Check sheet for the modelled part. Datum: model origin and axes. Units: mm. Face numbers are marked on the shaded views. A direction names the side the tool comes from. Coordinates: 2 decimals unless noted, no trailing zeros. Order: outer loops, then holes, each group sorted by start corner. A loop starts at its lowest first (then second) coordinate and runs counter-clockwise, first axis right, second up.
1. Cross-section at D-D (z = 1.75). Enter the section's corners in (x, y), then the cut area to 3 significant figures.
2. Gauge pin test, flat ends, axial feed: pin 1 Ø1 at (x, z) = (1, 3.5) entering from -Y; pin 2 Ø3 at (x, y) = (0, 0) entering from +Z; pin 3 Ø4 at (y, z) = (0.5, 3) entering from +X; pin 4 Ø3 at (x, z) = (-3, -2) entering from +Y. Record the tip position at first contact, or that the pin passes through.
3. Set-up check for the marked faces 4, 5 and 6: record each of +Z, -Z, +X, -X, +Y, -Y from which the full face is reachable in a straight line by a thin tool's end or side.
4. Thickness scan on line 1 (Y direction, x = 0, z = -0.5); line 2 (Z direction, x = -3.5, y = -1.5); line 3 (Y direction, x = -4, z = 3.5). Record the ranges inside material, lowest first.
5. Cross-section at C-C (z = -1.5). Enter the section's corners in (x, y), then the cut area to 3 significant figures.
6. Cross-section at A-A (x = 0). Enter the section's corners in (y, z).
7. Draft check along Y on the marked faces 1, 2 and 3. Enter one of: released by +Y, released by -Y, zero draft, split by the parting line, or undercut.
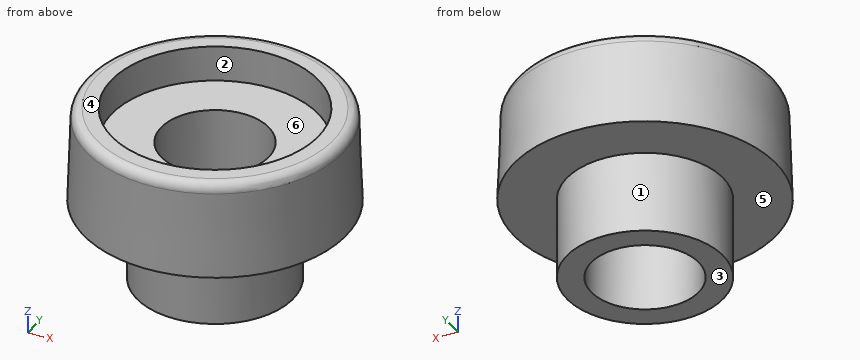
```python
from build123d import *

# Parameters (mm, degrees)
ESQUISSE1_R             = 6.45
ESQUISSE1_R_2           = 5.15
BOSS_EXTRU_1_DEPTH      = 4.7
BOSS_EXTRU_1_DRAFT      = 2
ESQUISSE2_R             = 6.285872383
ESQUISSE2_R_2           = 2.65
BOSS_EXTRU_2_DEPTH      = 4.7
CONG_1_R                = 0.5
ESQUISSE4_R             = 5.080745256
ENL_V_MAT_EXTRU_1_DEPTH = 1.75
ESQUISSE3_R             = 3.85
ESQUISSE3_R_2           = 2.65
BOSS_EXTRU_8_DEPTH      = 4


with BuildPart() as part:
    # Esquisse1 → Boss.-Extru.1 (with draft: the straight prism first)
    with BuildSketch(Plane.XY):
        Circle(ESQUISSE1_R)
        Circle(ESQUISSE1_R_2, mode=Mode.SUBTRACT)
    extrude(amount=BOSS_EXTRU_1_DEPTH)
    # Boss.-Extru.1: the draft: its side faces are tilted about the plane it starts from
    boss_extru_1_sides = [part.faces().sort_by_distance(p)[0] for p in [
        (-6.45, 0, 2.35),
        (-5.15, 0, 2.35),
    ]]
    draft(boss_extru_1_sides, Plane.XY, BOSS_EXTRU_1_DRAFT)

    # Esquisse2 → Boss.-Extru.2 (add)
    with BuildSketch(Plane.XY.offset(4.7)):
        Circle(ESQUISSE2_R)
        Circle(ESQUISSE2_R_2, mode=Mode.SUBTRACT)
    extrude(amount=-BOSS_EXTRU_2_DEPTH)

    # Congé1
    cong_1_edges = [part.edges().sort_by_distance(p)[0] for p in [
        (-6.285872383, 0, 4.7),
    ]]
    fillet(cong_1_edges, radius=CONG_1_R)

    # Esquisse4 → Enlèv. mat.-Extru.1 (cut)
    with BuildSketch(Plane.XY.offset(4.7)):
        Circle(ESQUISSE4_R)
    extrude(amount=-ENL_V_MAT_EXTRU_1_DEPTH, mode=Mode.SUBTRACT)

    # Esquisse3 → Boss.-Extru.8 (add)
    with BuildSketch(Plane(origin=(0, 0, 0), x_dir=(-1, 0, 0), z_dir=(0, 0, -1))):
        with Locations(Location((0, 0, 0), (0, 0, 180))):
            Circle(ESQUISSE3_R)
        with Locations(Location((0, 0, 0), (0, 0, 180))):
            Circle(ESQUISSE3_R_2, mode=Mode.SUBTRACT)
    extrude(amount=BOSS_EXTRU_8_DEPTH)


solid = part.part
```
Data:
1. outline: circle Ø12.78 at (0, 0); hole circle Ø5.3 at (0, 0)
1. area: 106 mm2
2. pin 1: stops at y = -6.31
2. pin 2: passes through
2. pin 3: stops at x = 6.41
2. pin 4: stops at y = 3.55
3. face 4: +Z, +X, -X, +Y, -Y
3. face 5: -Z
3. face 6: +Z
4. line 1: y = -3.85 to -2.65, 2.65 to 3.85
4. line 2: z = -4 to 2.95
4. line 3: y = -4.9 to -3.13, 3.13 to 4.9
5. outline: circle Ø7.7 at (0, 0); hole circle Ø5.3 at (0, 0)
5. area: 24.5 mm2
6. outline: (-6.45, 0) - (-3.85, 0) - (-3.85, -4) - (-2.65, -4) - (-2.65, 2.95) - (-5.08, 2.95) - (-5.08, 4.7) - (-5.8, 4.7) arc R0.5 ccw to (-6.3, 4.22) - close; (2.65, -4) - (3.85, -4) - (3.85, 0) - (6.45, 0) - (6.3, 4.22) arc R0.5 ccw to (5.8, 4.7) - (5.08, 4.7) - (5.08, 2.95) - (2.65, 2.95) - close
7. face 1: split by the parting line
7. face 2: undercut
7. face 3: zero draft
